Geometry: final body of the model. Coordinates: model frame, mm. Round coordinates to 2 decimals unless told otherwise and drop trailing zeros. Write each loop counter-clockwise with the first axis right and the second up, starting at its lowest first coordinate (ties: lowest second). Pieces come first, ordered by that corner, then holes. Notation, with made-up numbers: (11.25, 32) -> (66.25, 32) arc R18 ccw to (66.25, 40) -> close; hole circle Ø8 at (66.25, -12.5). An arc over 180 degrees is marked (long way). Use one line per item in the form item = value. Start each with the question number.
1. Line query: L1, parallel to Y at x = 0, z = 4; L2, parallel to Z at x = 1, y = -20; L3, parallel to Y at x = 0, z = -5. Output: solid intervals per line, ascending.
2. Cut plane A-A, the plane z = 55.5. Return the cut outline in (x, y).
3. Pin query (flat end, axial travel): pin 1 Ø4 at (y, z) = (-19, 91.5) entering from +X; pin 2 Ø3 at (x, z) = (-4.5, 252) entering from +Y; pin 3 Ø5 at (x, y) = (9.5, -9) entering from +Z. Return the tip coordinate at first contact, or that it passes through.
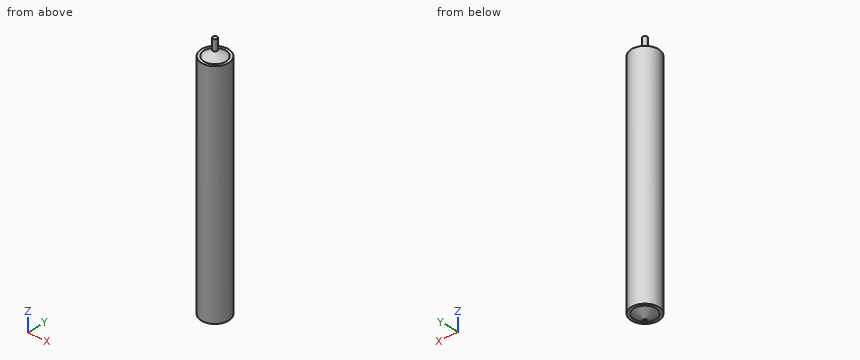
```python
from build123d import *

# Parameters (mm, degrees)
SCHIZZO1_R                   = 25
ESTRUSIONE_ESTRUSIONE1_DEPTH = 420
SCHIZZO5_R                   = 4
SCHIZZO4_R                   = 20
SCHIZZO9_R                   = 4
ESTRUSIONE_ESTRUSIONE2_DEPTH = 20
SCHIZZO12_R                  = 2.5
TAGLIO_ESTRUSIONE2_DEPTH     = 25


with BuildPart() as part:
    # Schizzo1 → Estrusione-Estrusione1 (new body)
    with BuildSketch(Plane.XY):
        Circle(SCHIZZO1_R)
    extrude(amount=ESTRUSIONE_ESTRUSIONE1_DEPTH)

    # Schizzo5 → Loft2 section 0
    with BuildSketch(Plane.XY.offset(430)):
        Circle(SCHIZZO5_R)
    # Schizzo4 → Loft2 section 1
    with BuildSketch(Plane.XY.offset(420)):
        Circle(SCHIZZO4_R)
    loft()

    # Schizzo9 → Estrusione-Estrusione2 (add)
    with BuildSketch(Plane.XY.offset(430)):
        with Locations(Location((0, 0, 0), (0, 0, 180))):
            Circle(SCHIZZO9_R)
    extrude(amount=ESTRUSIONE_ESTRUSIONE2_DEPTH)

    # Loft3: read off the stored shape, not the designer's step
    # Loft3: loft between two sections, ruled curve by curve
    loft3_from = [
        Edge.make_bspline([(-8.012098274, 18.325017906, 0), (28.637937538, 34.349214454, 0), (44.662134086, -2.300821358, 0), (8.012098274, -18.325017906, 0), (-28.637937538, -34.349214454, 0), (-44.662134086, 2.300821358, 0), (-8.012098274, 18.325017906, 0)], [0, 0, 0, 0, 0.5, 0.5, 0.5, 1, 1, 1, 1], 3, [1, 0.333333333, 0.333333333, 1, 0.333333333, 0.333333333, 1]),
    ]
    loft3_to = [
        Edge.make_bspline([(-0.355363052, 2.474614536, -10), (4.59386602, 3.18534064, -10), (5.304592124, -1.763888432, -10), (0.355363052, -2.474614536, -10), (-4.59386602, -3.18534064, -10), (-5.304592124, 1.763888432, -10), (-0.355363052, 2.474614536, -10)], [0, 0, 0, 0, 0.5, 0.5, 0.5, 1, 1, 1, 1], 3, [1, 0.333333333, 0.333333333, 1, 0.333333333, 0.333333333, 1]),
    ]
    loft3 = Solid(Shell([*[Face.make_surface_from_curves(loft3_from[k], loft3_to[k]) for k in range(1)], Face(Wire(loft3_from)), Face(Wire(loft3_to))]))
    add(loft3)

    # Schizzo12 → Taglio-Estrusione2 (cut)
    with BuildSketch(Plane(origin=(0, 0, -10), x_dir=(-1, 0, 0), z_dir=(0, 0, -1))):
        Circle(SCHIZZO12_R)
    extrude(amount=-TAGLIO_ESTRUSIONE2_DEPTH, mode=Mode.SUBTRACT)


solid = part.part
```
Outcome:
q1.L1 = -25 to -2.5, 2.5 to 25
q1.L2 = 0 to 420
q1.L3 = -11.21 to -2.5, 2.5 to 11.21
q2.outline = circle Ø50 at (0, 0)
q3.pin_1 = 18.33
q3.pin_2 = 24.82
q3.pin_3 = 425.88
